The drawing under review shows one solid part. Ordinate dimensions are in mm from its lowest x, y, z. A direction names the side the tool comes from. Coordinates: 2 decimals unless noted, no trailing zeros. Write each loop counter-clockwise with the first axis right and the second up, starting at its lowest first coordinate (ties: lowest second). Pieces come first, ordered by that corner, then holes.
Q1. Mouldability with a two-part tool opening along Z and no side actions: class the marked faces 1, 2 and 3 as pulls with the +Z half, pulls with the -Z half, needs draft (parallel to the pull), parting line crosses it, or undercut.
Q2. Machinability: for the marked faces 4, 5 and 6, which of the approach directions +Z, -Z, +X, -X, +Y, -Y give a long, thin tool a straight path to every point of the face, cutting with its end or side? Answer none if there is none.
Q3. Insertion check: pin 1 (8 mm diameter, centred on y = 35.5, z = 22, fed in from +X); pin 2 (5.5 mm diameter, centred on y = 5.08, z = 14.224, fed in from +X); pin 3 (12 mm diameter, centred on x = 11.5, z = 18, fed in from +Y) (1 decimal); pin 4 (2 mm diameter, centred on x = 17, z = 4.5, fed in from +Y). Each pin has a flat end and moves straight along its axis. Give the tip position at first contact, or say it passes through.
Q4. For probe 1 along Y at (x, z) = (23.75, 13.75) (1 decimal); probe 2 along X at (y, z) = (10, 6) (1 decimal); probe 3 along Y at (x, z) = (8, 5), list the stretches that pass through material, from the lowest coordinate up.
Q5. Take a section at A-A (z = 12.5). State how many separate pieces and enclosed holes the cut face has.
Q6. Take a section at B-B (y = 37). Give the boundary of the cut face in (x, z).
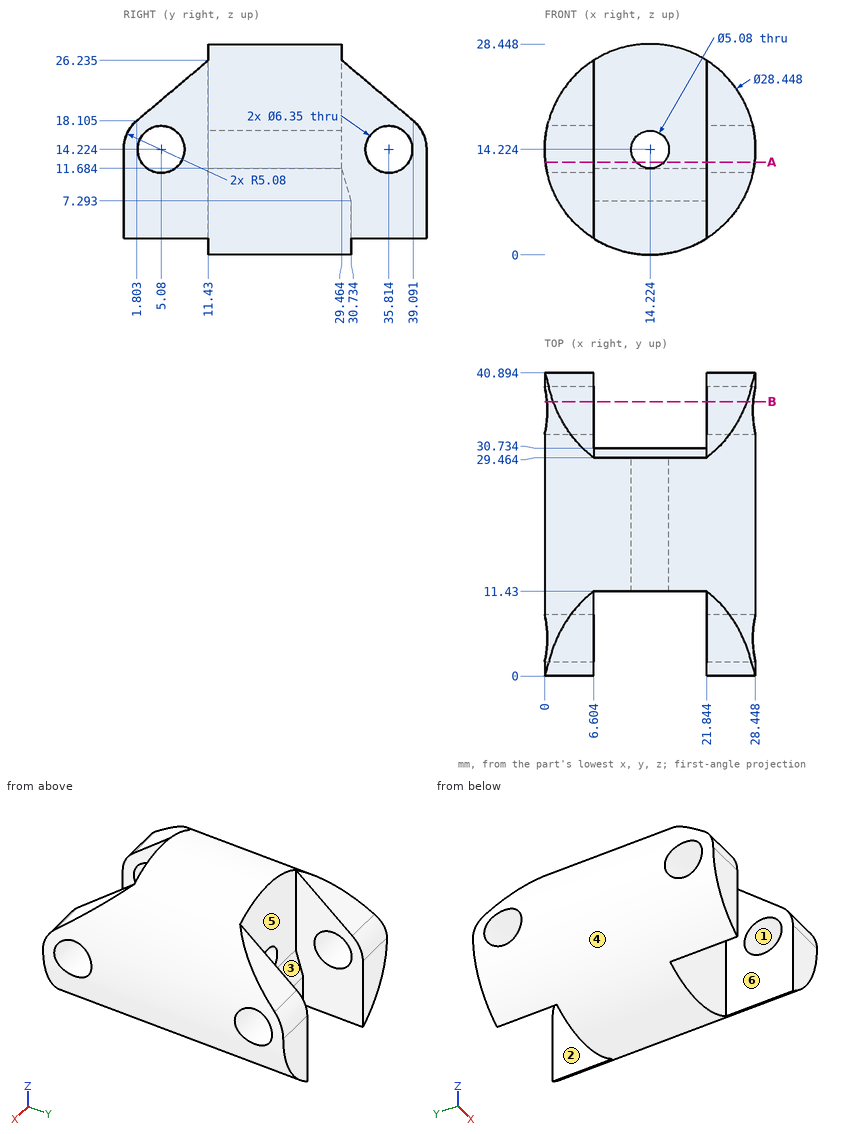
Response:
1. face 1: undercut
1. face 2: needs draft
1. face 3: pulls with the +Z half
2. face 4: +Y, -Y
2. face 5: +Z, +Y
2. face 6: +Z, -Z, -Y
3. pin 1: stops at x = 27.94
3. pin 2: passes through
3. pin 3: stops at y = 40.9
3. pin 4: stops at y = 30.73
4. probe 1: y = 0 to 1.9, 8.2 to 32.7, 39 to 40.9
4. probe 2: x = 2.6 to 6.6, 21.8 to 25.8
4. probe 3: y = 11.43 to 30.73
5. separate pieces: 6
5. enclosed holes: 0
6. outline: (0.31, 11.28) arc R14.22 ccw to (6.6, 2.21) - (6.6, 11.28) - close; (0.31, 17.17) - (6.6, 17.17) - (6.6, 19.87) - (1.17, 19.87) arc R14.22 ccw to start; (21.84, 2.21) arc R14.22 ccw to (28.14, 11.28) - (21.84, 11.28) - close; (21.84, 17.17) - (28.14, 17.17) arc R14.22 ccw to (27.28, 19.87) - (21.84, 19.87) - close
